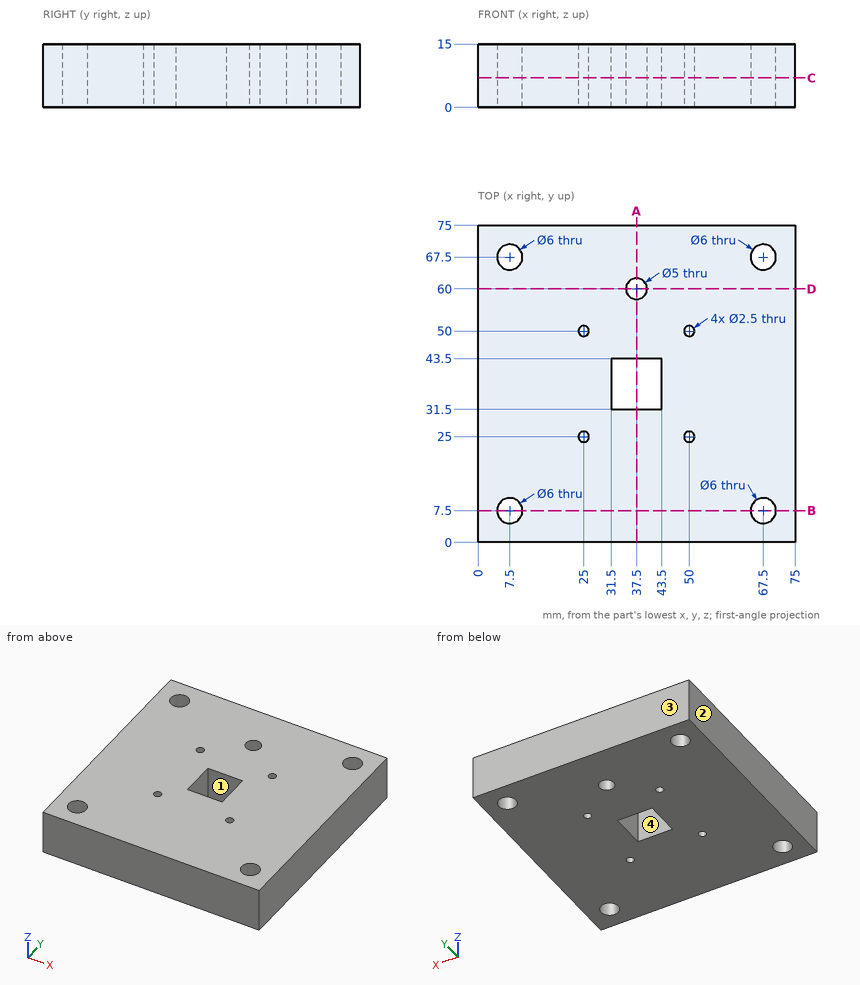
Drawing for the job (mm, zero at the part's lowest x, y, z). Round coordinates to 2 decimals unless told otherwise and drop trailing zeros. Write each loop counter-clockwise with the first axis right and the second up, starting at its lowest first coordinate (ties: lowest second). Pieces come first, ordered by that corner, then holes. Notation, with made-up numbers: M -14.5,63.25 L 41.5,63.25 A18 cw 41.5,87.25 Z; hole C -22,-5.75 d1. An arc over 180 degrees is marked long. One line per question, with ' | ' between items.
1. Probe L1, parallel to Y at x = 7.5, z = 8.25; L2, parallel to Y at x = 50, z = 3.75; L3, parallel to X at y = 34, z = 8. List the from-to ranges inside material, lowest first. Write a range as from..to.
Working result:
L1: 0..4.5, 10.5..64.5, 70.5..75 | L2: 0..23.75, 26.25..48.75, 51.25..75 | L3: 0..31.5, 43.5..75
2. Cut at A-A on x = 37.5. Write the cut outline in (y, z), and give its area (3 significant figures).
Working result:
outline: M 0,0 L 31.5,0 L 31.5,15 L 0,15 Z; M 43.5,0 L 57.5,0 L 57.5,15 L 43.5,15 Z; M 62.5,0 L 75,0 L 75,15 L 62.5,15 Z | area: 870 mm2
3. Cut at B-B on y = 7.5. Write the cut outline in (x, z).
Working result:
outline: M 0,0 L 4.5,0 L 4.5,15 L 0,15 Z; M 10.5,0 L 64.5,0 L 64.5,15 L 10.5,15 Z; M 70.5,0 L 75,0 L 75,15 L 70.5,15 Z
4. Pin check, flat tip, straight feed: pin 1 Ø2 at (x, y) = (55, 63.5) entering from -Z. Stop position of the tip, or through.
Working result:
pin 1: z = 0
5. Cut at D-D on y = 60. Write the cut outline in (x, z), and give its area (3 significant figures).
Working result:
outline: M 0,0 L 35,0 L 35,15 L 0,15 Z; M 40,0 L 75,0 L 75,15 L 40,15 Z | area: 1,050 mm2
6. Mould opens along Y. For the marked faces 1, 2, 3 and 4 say: pulls with the +Y half, pulls with the -Y half, needs draft (parallel to the pull), parting line crosses it, or undercut.
Working result:
face 1: undercut | face 2: needs draft | face 3: pulls with the +Y half | face 4: undercut
7. Cut at C-C on z = 7. Count the separate pieces of the cut face and the enclosed holes in it, and give its area (3 significant figures).
Working result:
separate pieces: 1 | enclosed holes: 10 | area: 5,330 mm2
